Autodesk Inventor part; units mm, degrees
ref_plane "YZ Plane" through (0, 0, 0) normal (1, 0, 0) x (0, 1, 0)
ref_plane "XZ Plane" through (0, 0, 0) normal (0, 1, 0) x (-1, 0, 0)
ref_plane "XY Plane" through (0, 0, 0) normal (0, 0, 1) x (1, 0, 0)
sketch "Skizze1" plane through (0, 0, 0) normal (0, 1, 0) x (-1, 0, 0)
  line L0 (0, 0) -> (0, -15)
  line L1 (0, -15) -> (5, -15)
  line L2 (5, -15) -> (10, -15) construction
  line L3 (10, -15) -> (15, -15)
  line L4 (15, -15) -> (15, 0)
  line L5 (15, 0) -> (10, 0)
  line L6 (10, 0) -> (5, 0) construction
  line L7 (5, 0) -> (0, 0)
  line L8 (0, -7.5) -> (0, -5.25) construction
  line L9 (0, -5.25) -> (0, -9.75) construction
  line L10 (0, -9.75) -> (9.7, -9.75) construction
  line L11 (0, -5.25) -> (9.7, -5.25) construction
  line L12 (15, -7.5) -> (15, -3.9) construction
  line L13 (15, -3.9) -> (15, -11.4) construction
  line L14 (15, -11.4) -> (9.7, -11.4) construction
  line L15 (9.7, -11.4) -> (9.7, -9.75) construction
  line L16 (15, -3.9) -> (9.7, -3.9) construction
  line L17 (9.7, -3.9) -> (9.7, -5.25) construction
  line L18 (10, 0) -> (8.5, -2.5981)
  line L19 (10, 0) -> (13, 0) construction
  line L20 (5, 0) -> (6.5, -2.5981)
  line L21 (5, 0) -> (8, 0) construction
  line L22 (6.5, -2.5981) -> (8.5, -2.5981)
  line L23 (10, -15) -> (8.5, -12.4019)
  line L24 (10, -15) -> (13, -15) construction
  line L25 (5, -15) -> (6.5, -12.4019)
  line L26 (5, -15) -> (8, -15) construction
  line L27 (6.5, -12.4019) -> (8.5, -12.4019)
  dimension "d0" = 15
  dimension "d1" = 5
  dimension "d2" = 5
  dimension "d3" = 5
  dimension "d4" = 15
  dimension "d5" = 5
  dimension "d6" = 5
  dimension "d7" = 2.25
  dimension "d8" = 4.5
  dimension "d9" = 9.7
  dimension "d10" = 9.7
  dimension "d11" = 3.6
  dimension "d12" = 7.5
  dimension "d13" = 5.3
  dimension "d14" = 3
  dimension "d15" = 120
  dimension "d16" = 3
  dimension "d17" = 60
  dimension "d18" = 3
  dimension "d19" = 120
  dimension "d20" = 3
  dimension "d21" = 60
extrude "Extrusion1" add sketch "Skizze1" along normal blind 300
sketch "Skizze2" plane through (0, 0, 0) normal (1, 0, 0) x (0, 0, -1)
  line L0 (15, 300) -> (0, 300) construction
  line L1 (7.5, 300) -> (7.5, 270) construction
  line L2 (7.5, 270) -> (7.5, 210) construction
  line L3 (7.5, 210) -> (7.5, 150) construction
  line L4 (7.5, 150) -> (7.5, 90) construction
  line L5 (7.5, 90) -> (7.5, 30) construction
  point P0 (0, 0)
  dimension "d25" = 30
  dimension "d26" = 60
  dimension "d27" = 60
  dimension "d28" = 60
  dimension "d29" = 60
hole "Bohrung1" at (0, 270, -7.5) at (0, 210, -7.5) at (0, 150, -7.5) at (0, 90, -7.5) at (0, 30, -7.5) direction (-1, 0, 0) diameter 4.5 end through all counterbore diameter 7.5 counterbore depth 5.3
chamfer "Fase1" distance 1 angle 45 4 edges at (0, 150, -15) (0, 150, 0) (-15, 150, -15) (-15, 150, 0)
chamfer "Fase2" distance 0.1 angle 45 5 edges at (0, 270, -3.75) (0, 210, -3.75) (0, 150, -3.75) (0, 90, -3.75) (0, 30, -3.75)
properties part number "Linearführung" material "Edelstahl"
Part model, mm, in its own coordinate system. A direction names the side the tool comes from. Give positions to 0.01 mm unless a question says otherwise; leave off trailing zeros. Loops run counter-clockwise (first coordinate to the right, second up) from the corner with the lowest first, then second, coordinate; pieces in that order, holes last.
(1) Pull direction Y, two halves, no side cores. Call faces 3 (the flat face through (-7, 0, -7)), 4 (the flat face through (-7, 300, -7)), 5 (the flat face through (-15, 148, -6)), 6 (the flat face through (-5.3, 92, -9)): pulls with the +Y half, pulls with the -Y half, needs draft (parallel to the pull), parting line crosses it, or undercut.
Return value:
face 3: pulls with the -Y half
face 4: pulls with the +Y half
face 5: needs draft
face 6: undercut
(2) Band-saw the part on A-A (y = 185). Write the cut outline in (x, z).
Return value:
outline: (-15, -14) - (-14, -15) - (-10, -15) - (-8.5, -12.4) - (-6.5, -12.4) - (-5, -15) - (-1, -15) - (0, -14) - (0, -1) - (-1, 0) - (-5, 0) - (-6.5, -2.6) - (-8.5, -2.6) - (-10, 0) - (-14, 0) - (-15, -1) - close
(3) 3-axis set-ups, long thin cutter, end or side, ignore diameter. For faces 1 (the flat face through (-5.3, 152, -9)), 2 (the flat face through (0, 148, -12)): which of +Z, -Z, +X, -X, +Y, -Y reach the whole face in a straight line?
Return value:
face 1: +X
face 2: +Z, -Z, +X, +Y, -Y
(4) Pin check, flat tips, straight feed: pin 1 (6 mm diameter, centred on y = 29.5, z = -7, fed in from +X); pin 2 (6 mm diameter, centred on y = 150, z = -7.5, fed in from -X); pin 3 (4 mm diameter, centred on x = -7.5, y = 99.5, fed in from -Z); pin 4 (1.6 mm diameter, centred on x = -8, y = 209, fed in from -Z). Stop position of each tip, or through.
Return value:
pin 1: stops at x = -5.3
pin 2: stops at x = -15
pin 3: stops at z = -14.13
pin 4: stops at z = -12.92
(5) Drill centre lines: line 1 along Y through (x, z) = (-12.5, -7.5); line 2 along Y through (x, z) = (-2.7, -7.5); line 3 along Z through (x, y) = (-3.7, 30). Where is each one in solid material? Low to high.
Return value:
line 1: y = 0 to 27.75, 32.25 to 87.75, 92.25 to 147.75, 152.25 to 207.75, 212.25 to 267.75, 272.25 to 300
line 2: y = 0 to 26.25, 33.75 to 86.25, 93.75 to 146.25, 153.75 to 206.25, 213.75 to 266.25, 273.75 to 300
line 3: z = -15 to -11.25, -3.75 to 0
(6) Band-saw the part on B-B (z = -7.5). Count the separate pieces of the cut face and the enclosed holes in it, and give its area (3 significant figures).
Return value:
separate pieces: 6
enclosed holes: 0
area: 4,080 mm2
